Build history of the part. All positions in model axes, mm. Face numbers are marked on the shaded views. A direction names the side the tool comes from. Round coordinates to 2 decimals unless told otherwise and drop trailing zeros. Order: outer loops, then holes, each group sorted by start corner. A loop starts at its lowest first (then second) coordinate and runs counter-clockwise, first axis right, second up. Notation, with made-up numbers: M -21,-32 L -6,-32 A11 cw -6,-17 Z; hole C 77.5,-0.75 d8. An arc over 180 degrees is marked long. Use CSV: the item, a comma, the result in double quotes.
from build123d import *

# Parameters (mm, degrees)
EXTRUDE1_DEPTH     = 19.685
CHAMFER1_SIZE      = 3.302
FILLET1_R          = 0.762
SKETCH2_W          = 17.907
SKETCH2_H          = 2.54
EXTRUDE2_DEPTH     = 7.493
SKETCH4_W          = 17.907
SKETCH4_H          = 2.54
EXTRUDE3_DEPTH     = 7.493
FILLET2_R          = 0.762
EXTRUDE4_DEPTH     = 36.35375
SKETCH10_R         = 2.159
CUT_EXTRUDE1_DEPTH = 36.35375
RIB2_START         = -0.6985
RIB2_DEPTH         = 1.397
RIB3_START         = -0.6985
RIB3_DEPTH         = 1.397
SKETCH16_R         = 5.0165
EXTRUDE5_DEPTH     = 1.651
SKETCH18_R         = 4.953
EXTRUDE6_DEPTH     = 0.127
SKETCH19_R         = 2.159
CUT_EXTRUDE2_DEPTH = 59.305619446
SKETCH20_R         = 2.8575
SKETCH20_R_2       = 1.27
EXTRUDE7_DEPTH     = 4.064
SKETCH22_W         = 5.715
SKETCH22_H         = 3.175
EXTRUDE8_DEPTH     = 1.905
SKETCH24_R         = 0.635


with BuildPart() as part:
    # Sketch1 → Extrude1 (new body)
    with BuildSketch(Plane.XY):
        Polygon((0, 0), (39.6875, 0), (39.6875, 31.59125), (20.6375, 35.56), (0, 35.56), align=None)
    extrude(amount=EXTRUDE1_DEPTH)

    # Chamfer1
    chamfer1_edges = [part.edges().sort_by_distance(p)[0] for p in [
        (0, 35.56, 9.8425),
    ]]
    chamfer(chamfer1_edges, length=CHAMFER1_SIZE)

    # Fillet1
    fillet1_edges = [part.edges().sort_by_distance(p)[0] for p in [
        (19.84375, 0, 0),
        (19.84375, 0, 19.685),
        (39.6875, 0, 9.8425),
        (0, 0, 9.8425),
    ]]
    fillet(fillet1_edges, radius=FILLET1_R)

    # Sketch2 → Extrude2 (add)
    with BuildSketch(Plane(origin=(39.6875, 0, 0), x_dir=(0, 0, -1), z_dir=(1, 0, 0))):
        with Locations((-9.8425, 26.76525)):
            Rectangle(SKETCH2_W, SKETCH2_H)
    extrude(amount=EXTRUDE2_DEPTH)

    # Sketch4 → Extrude3 (add)
    with BuildSketch(Plane.ZY):
        with Locations((9.8425, 26.76652)):
            Rectangle(SKETCH4_W, SKETCH4_H)
    extrude(amount=EXTRUDE3_DEPTH)

    # Fillet2
    fillet2_edges = [part.edges().sort_by_distance(p)[0] for p in [
        (47.1805, 26.76525, 18.796),
        (47.1805, 26.76525, 0.889),
        (-7.493, 26.76652, 0.889),
        (-7.493, 26.76652, 18.796),
    ]]
    fillet(fillet2_edges, radius=FILLET2_R)

    # Sketch5 → Extrude4 (add)
    with BuildSketch(Plane(origin=(0, 0, 0), x_dir=(1, 0, 0), z_dir=(0, 1, 0))):
        with BuildLine():
            Line((1.143, -0.837535442), (20.828, -0.837535442))
            Line((20.828, -0.837535442), (20.828, -7.022435442))
            ThreePointArc((20.828, -7.022435442), (18.034, -9.816435442), (20.828, -12.610435442))
            Line((20.828, -12.610435442), (20.828, -18.795335442))
            Line((20.828, -18.795335442), (1.143, -18.795335442))
            Line((1.143, -18.795335442), (1.143, -0.837535442))
        make_face()
    extrude(amount=EXTRUDE4_DEPTH)

    # Sketch9 → Loft1 section 0
    with BuildSketch(Plane(origin=(7.958631448, 38.201430948, 0), x_dir=(-0.9789804197376049, 0.20395425411200233, 0), z_dir=(0.20395425411200233, 0.9789804197376049, 0))):
        with BuildLine():
            Line((-29.108115578, 18.877249077), (-13.970346323, 18.877249077))
            Line((-13.970346323, 18.877249077), (-13.970346323, 11.936940395))
            ThreePointArc((-13.970346323, 11.936940395), (-11.890798187, 9.857392259), (-13.970346323, 7.777844123))
            Line((-13.970346323, 7.777844123), (-13.970346323, 0.837535442))
            Line((-13.970346323, 0.837535442), (-29.108115578, 0.837535442))
            Line((-29.108115578, 0.837535442), (-29.108115578, 18.877249077))
        make_face()
    # Sketch7 → Loft1 section 1
    with BuildSketch(Plane(origin=(0, 36.35375, 0), x_dir=(-1, 0, 0), z_dir=(0, 1, 0))):
        with BuildLine():
            Line((-21.844, 0.837535442), (-34.544, 0.837535442))
            Line((-34.544, 0.837535442), (-34.544, 18.795335442))
            Line((-34.544, 18.795335442), (-21.844, 18.795335442))
            Line((-21.844, 18.795335442), (-21.844, 11.911935442))
            ThreePointArc((-21.844, 11.911935442), (-19.7485, 9.816435442), (-21.844, 7.720935442))
            Line((-21.844, 7.720935442), (-21.844, 0.837535442))
        make_face()
    loft()

    # Sketch10 → Cut-Extrude1 (cut)
    with BuildSketch(Plane(origin=(0, 28.03525, 0), x_dir=(-1, 0, 0), z_dir=(0, 1, 0))):
        with Locations(Location((-43.7515, 4.699, 0), (0, 0, 90))):
            Circle(SKETCH10_R)
        with Locations(Location((-43.7515, 14.986, 0), (0, 0, 90))):
            Circle(SKETCH10_R)
    extrude(amount=-CUT_EXTRUDE1_DEPTH, mode=Mode.SUBTRACT)

    # Rib2: read off the stored shape, not the designer's step
    # Rib2 outline → Rib2 (add)
    with BuildSketch(Plane.XY.offset(9.8425).offset(RIB2_START)):
        Polygon((43.622065389, 28.03525), (42.556674437, 29.225981064), (39.6875, 29.914582929), (39.6875, 28.03525), align=None)
    extrude(amount=RIB2_DEPTH)

    # Rib3: read off the stored shape, not the designer's step
    # Rib3 outline → Rib3 (add)
    with BuildSketch(Plane.XY.offset(9.8425).offset(RIB3_START)):
        Polygon((0, 29.585656003), (-3.58232689, 28.876779051), (-4.304067283, 28.03652), (0, 28.03652), align=None)
    extrude(amount=RIB3_DEPTH)

    # Sketch16 → Extrude5 (add)
    with BuildSketch(Plane(origin=(0, 36.35375, 0), x_dir=(-1, 0, 0), z_dir=(0, 1, 0))):
        with Locations(Location((-9.77846774, 9.8425, 0), (0, 0, 270))):
            Circle(SKETCH16_R)
    extrude(amount=EXTRUDE5_DEPTH)

    # Loft2: read off the stored shape, not the designer's step
    # Loft2: loft between two sections, ruled curve by curve
    loft2_from = [
        Edge.make_bspline([(10.784981125, 36.35375, 2.802082768), (-3.29585334, 36.35375, 0.789055998), (-5.308880109, 36.35375, 14.869890463), (8.771954355, 36.35375, 16.882917232), (22.85278882, 36.35375, 18.895944002), (24.865815589, 36.35375, 4.815109537), (10.784981125, 36.35375, 2.802082768)], [0, 0, 0, 0, 0.5, 0.5, 0.5, 1, 1, 1, 1], 3, [1, 0.333333333, 0.333333333, 1, 0.333333333, 0.333333333, 1]),
    ]
    loft2_to = [
        Edge.make_bspline([(9.491795646, 38.00475, 4.834197757), (-0.52480884, 38.00475, 5.407541944), (0.048535347, 38.00475, 15.424146431), (10.065139834, 38.00475, 14.850802243), (20.08174432, 38.00475, 14.277458056), (19.508400133, 38.00475, 4.260853569), (9.491795646, 38.00475, 4.834197757)], [0, 0, 0, 0, 0.5, 0.5, 0.5, 1, 1, 1, 1], 3, [1, 0.333333333, 0.333333333, 1, 0.333333333, 0.333333333, 1]),
    ]
    loft2 = Solid(Shell([*[Face.make_surface_from_curves(loft2_from[k], loft2_to[k]) for k in range(1)], Face(Wire(loft2_from)), Face(Wire(loft2_to))]))
    add(loft2)

    # Sketch18 → Extrude6 (add)
    with BuildSketch(Plane(origin=(0, 38.00475, 0), x_dir=(-1, 0, 0), z_dir=(0, 1, 0))):
        with Locations(Location((-9.77846774, 9.8425, 0), (0, 0, 90))):
            Circle(SKETCH18_R)
    extrude(amount=EXTRUDE6_DEPTH)

    # Sketch19 → Cut-Extrude2 (cut, through all)
    with BuildSketch(Plane(origin=(0, 28.03652, 0), x_dir=(-1, 0, 0), z_dir=(0, 1, 0))):
        with Locations(Location((4.064, 4.699, 0), (0, 0, 90))):
            Circle(SKETCH19_R)
        with Locations(Location((4.064, 14.986, 0), (0, 0, 90))):
            Circle(SKETCH19_R)
    extrude(amount=-CUT_EXTRUDE2_DEPTH, mode=Mode.SUBTRACT)

    # Sketch20 → Extrude7 (add)
    with BuildSketch(Plane(origin=(0, 38.13175, 0), x_dir=(-1, 0, 0), z_dir=(0, 1, 0))):
        with Locations(Location((-9.77846774, 9.8425, 0), (0, 0, 90))):
            Circle(SKETCH20_R)
        with Locations(Location((-9.77846774, 9.8425, 0), (0, 0, 90))):
            Circle(SKETCH20_R_2, mode=Mode.SUBTRACT)
    extrude(amount=EXTRUDE7_DEPTH)

    # Sketch22 → Extrude8 (add)
    with BuildSketch(Plane.ZY):
        with Locations((9.8425, 2.8575)):
            Rectangle(SKETCH22_W, SKETCH22_H)
    extrude(amount=EXTRUDE8_DEPTH)

    # Sketch21 → section 0 of loft3
    with BuildSketch(Plane.ZY, mode=Mode.PRIVATE) as loft3_s0:
        with BuildLine():
            Line((6.477, 4.953), (13.208, 4.953))
            Line((13.208, 4.953), (13.208, 0.762))
            Line((13.208, 0.762), (6.477, 0.762))
            Line((6.477, 0.762), (6.477, 4.953))
        make_face()
    # loft up to a face of the part (loft3)
    loft([loft3_s0.sketch, part.faces().sort_by_distance((-1.905, 2.8575, 9.8425))[0]])

    # Sweep3: sweep along a path in Sketch23
    with BuildLine(Plane.XY.offset(9.8425)) as sweep3_path:
        ThreePointArc((-1.905, 2.946484605), (-3.908218654, 2.753050744), (-5.763136487, 1.972293764))
    # Sketch24 → Sweep3 (sweep)
    with BuildSketch(Plane.ZY.offset(1.905)):
        with Locations((9.8425, 2.946484605)):
            Circle(SKETCH24_R)
        with Locations((11.23883905, 2.946484605)):
            Circle(SKETCH24_R)
        with Locations((8.466018651, 2.946484605)):
            Circle(SKETCH24_R)
    sweep(path=sweep3_path.line)


solid = part.part
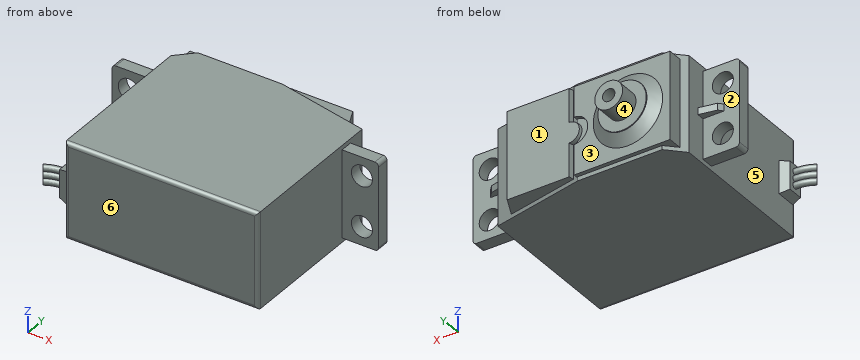
(1) Wall check: line 1 (X direction, y = 28, z = 3); line 2 (Y direction, x = 27, z = 9.75); line 3 (X direction, y = 22.5, z = 4.75). Give the ranges that are in metal, low to high. Write a range as from..to.
Answer block:
line 1,"x = -7.49..-5.4, -2.73..42.42, 45.08..47.18"
line 2,"y = 0..36.35"
line 3,"x = 0..39.69"
(2) Tool access for the marked faces 1, 2 and 3: list every direction of +Z, -Z, +X, -X, +Y, -Y with a clear straight run to the whole face (end or side of a thin tool).
Answer block:
face 1,"+Z, -Z, +X, +Y"
face 2,"-X, +Y"
face 3,"+Y"
(3) Cut at B-B, the plane y = 17. Give the cut face in (x, z) (1 decimal).
Answer block:
outline,"M 0,0 L 39.7,0 L 39.7,19.7 L 0,19.7 Z"
(4) Drop flat-ended pins along their axis: pin 1 (6 mm diameter, centred on x = -2.5, z = 13, fed in from +Y); pin 2 (1.3 mm diameter, centred on x = 19.5, z = 9.5, fed in from +Y); pin 3 (2 mm diameter, centred on x = -4.5, z = 8, fed in from -Y). Give the stop position or say it passes through.
Answer block:
pin 1,"stops at y = 32.76"
pin 2,"stops at y = 36.35"
pin 3,"stops at y = 1.45"
(5) Cut at A-A, the plane z = 15.75. Count the separate pieces of the cut face and the enclosed holes in it, and give its area (3 significant figures).
Answer block:
separate pieces,"3"
enclosed holes,"0"
area,"1,440 mm²"
(6) Two-plate mould, pull along Y, no slides. Class the marked faces 4, 5 and 6: released by +Y, released by -Y, zero draft, split by the parting line, or undercut.
Answer block:
face 4,"zero draft"
face 5,"undercut"
face 6,"released by -Y"
